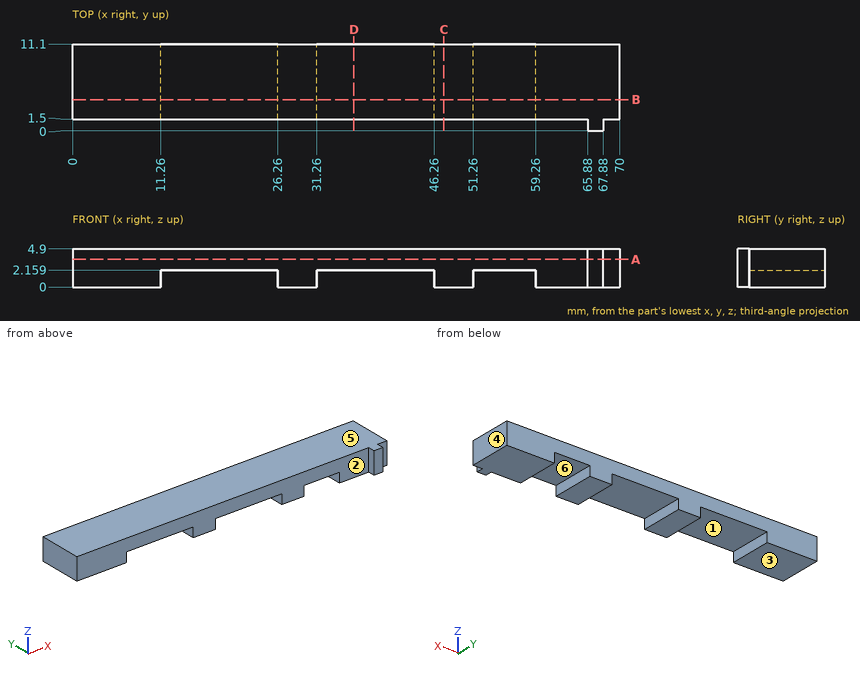
Drawing for the job (mm, zero at the part's lowest x, y, z). A direction names the side the tool comes from. Give positions to 0.01 mm unless a question says otherwise; leave off trailing zeros. Order: outer loops, then holes, each group sorted by start corner. A loop starts at its lowest first (then second) coordinate and runs counter-clockwise, first axis right, second up. Notation, with made-up numbers: (-34.75, 44.25) - (8.25, 44.25) arc R10 cw to (8.25, 58.25) - close; hole circle Ø8 at (7, -11). An arc over 180 degrees is marked (long way). Write item = value, one per line. Start each with the question number.
1. Two-plate mould, pull along X, no slides. Class the marked faces 4, 5 and 6: pulls with the +X half, pulls with the -X half, needs draft (parallel to the pull), parting line crosses it, or undercut.
2. Which spindle directions (+Z, -Z, +X, -X, +Y, -Y) get a long thin tool onto all of the face, cutting with end or side? Do the marked faces 1, 2 and 3. Say none if no direction does.
3. Cut at D-D, the plane x = 36. List the corners of the cut face in (y, z), and give its area (3 significant figures).
4. Cut at A-A, the plane z = 3.55. List the corners of the cut face in (x, y), and give its area (3 significant figures).
5. Probe line 1 along X through (y, z) = (1.75, 1.75); line 2 along Y through (x, z) = (4.5, 2.95); line 3 along Z through (x, y) = (18, 6.25). List the from-to ranges inside material, lowest first.
6. Cut at C-C, the plane x = 47.5. List the corners of the cut face in (y, z).
7. Cut at B-B, the plane y = 4. List the corners of the cut face in (x, z), and give its area (3 significant figures).
8. Drop flat-ended pins along their axis: P1, Ø3, axis at x = 21.5, y = 7, coming from the -Z side; P2, Ø1.7, axis at y = 8.5, z = 1, coming from the -X side; P3, Ø1.6, axis at y = 0.5, z = 3, coming from the +X side; P4, Ø1.5, axis at x = 46.5, z = 3, coming from the -Y side. Give the stop position or say it passes through.
Taken from the geometry:
q1.face_4 = pulls with the +X half
q1.face_5 = needs draft
q1.face_6 = undercut
q2.face_1 = -Z, +Y, -Y
q2.face_2 = +Z, -Z, -X, -Y
q2.face_3 = -Z, +X, -X, +Y, -Y
q3.outline = (1.5, 2.16) - (11.1, 2.16) - (11.1, 4.9) - (1.5, 4.9) - close
q3.area = 26.3 mm²
q4.outline = (0, 1.5) - (65.88, 1.5) - (65.88, 0) - (67.88, 0) - (67.88, 1.5) - (70, 1.5) - (70, 11.1) - (0, 11.1) - close
q4.area = 675 mm²
q5.line_1 = 0 to 11.26, 26.26 to 31.26, 46.26 to 51.26, 59.26 to 70
q5.line_2 = 1.5 to 11.1
q5.line_3 = 2.16 to 4.9
q6.outline = (1.5, 0) - (11.1, 0) - (11.1, 4.9) - (1.5, 4.9) - close
q7.outline = (0, 0) - (11.26, 0) - (11.26, 2.16) - (26.26, 2.16) - (26.26, 0) - (31.26, 0) - (31.26, 2.16) - (46.26, 2.16) - (46.26, 0) - (51.26, 0) - (51.26, 2.16) - (59.26, 2.16) - (59.26, 0) - (70, 0) - (70, 4.9) - (0, 4.9) - close
q7.area = 261 mm²
q8.P1 = 2.16
q8.P2 = 0
q8.P3 = 67.88
q8.P4 = 1.5
